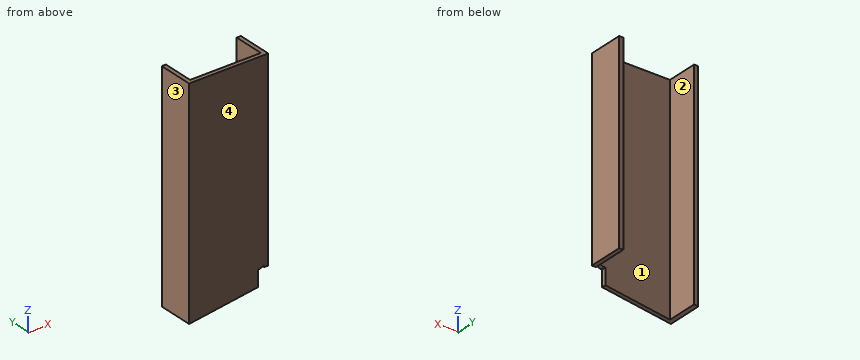
Autodesk Inventor part; units mm, degrees
ref_plane "XZ Plane" through (0, 0, 0) normal (0, 1, 0) x (-1, 0, 0)
ref_plane "XY Plane" through (0, 0, 0) normal (0, 0, 1) x (1, 0, 0)
sketch "Sketch1" plane through (0, 0, 0) normal (0, 0, 1) x (1, 0, 0)
  line L0 (10.7104, 9.7791) -> (42.7104, 9.7791)
  line L1 (42.7104, 9.7791) -> (42.7104, 24.7791)
  line L2 (10.7104, 9.7791) -> (10.7104, 24.7791)
  line L3 (8.7104, 24.7791) -> (8.7104, 7.7791)
  line L4 (8.7104, 7.7791) -> (44.7104, 7.7791)
  line L5 (44.7104, 7.7791) -> (44.7104, 24.7791)
  line L6 (8.7104, 24.7791) -> (10.7104, 24.7791)
  line L7 (42.7104, 24.7791) -> (44.7104, 24.7791)
  point P0 (0, 0)
  dimension "d0" = 32
  dimension "d1" = 15
  dimension "d2" = 15
  dimension "d3" = 2
extrude "Extrusion1" add sketch "Sketch1" along normal blind 100 and the other way blind 5
sketch "Sketch3" plane through (10.7104, 9.7791, 100) normal (0, 1, 0) x (1, 0, 0)
  line L0 (-2, 105) -> (-2, 0)
  line L1 (-2, 91.8971) -> (-2, 105)
  line L2 (32, 105) -> (34, 105)
  line L3 (34, 105) -> (-2, 91.8971)
  line L4 (-2, 105) -> (-2, 91.8971)
  line L5 (-2, 105) -> (34, 105)
  line L6 (0, 105) -> (0, 0)
  line L7 (0, 92.625) -> (0, 105)
  line L8 (34, 105) -> (-2, 99.9405)
  line L9 (34, 105) -> (70.3538, 105) construction
  line L10 (-2, 99.9405) -> (-2, 105)
  point P0 (-10.7104, 100)
  point P1 (-2, 99.9405)
  point P2 (0, 100.2216)
  dimension "d15" = 20
  dimension "d16" = 172
extrude "Extrusion4" cut sketch "Sketch3" along normal through all both and the other way through all contours L5 L6 L8 L0 | L5 L2 L8 L6
extrude "Extrusion5" cut sketch "Sketch3" along normal through all both and the other way through all contours L8 L6 L3 L0
ref_plane "Work Plane1" through (25.71, 0, 0) normal (1, 0, 0) x (0, 1, 0)
mirror "Mirror1" about plane through (25.71, 0, 0) normal (1, 0, 0) of "Extrusion5", "Extrusion4", "Extrusion1"
sketch "Sketch4" plane through (44.7104, 7.7791, 100) normal (1, 0, 0) x (0, 0, -1)
  line L0 (92.625, 2) -> (92.625, 17)
  line L1 (92.625, 17) -> (92.625, 2)
  line L2 (92.625, 2) -> (105, 2)
  line L3 (105, 17) -> (105, 0)
  line L4 (104.7189, 17) -> (0, 17)
  line L5 (105, 17) -> (93.3527, 17)
  line L6 (92.625, 2) -> (92.625, 0)
  line L7 (105, 0) -> (0, 0)
  line L8 (92.625, 0) -> (105, 0)
  line L9 (105, 0) -> (105, 2)
  line L10 (92.625, 17) -> (0, 17)
  line L11 (0, 0) -> (0, 17)
  line L12 (91.8971, 2) -> (0, 2)
  line L13 (0, 2) -> (91.8971, 2)
  point P0 (100, -7.7791)
  point P1 (95.3874, 17)
sketch "Sketch5" plane through (25.71, 0, 0) normal (1, 0, 0) x (0, 1, 0)
  line L0 (7.7791, 100) -> (24.7791, 100)
  line L1 (24.7791, 100) -> (9.7791, 100)
  line L2 (7.7791, 7.375) -> (9.7791, 7.375)
  line L3 (9.7791, 100) -> (9.7791, 7.375)
  line L4 (9.7791, 7.375) -> (24.7791, 7.375)
  line L5 (24.7791, 7.375) -> (24.7791, 100)
  line L6 (9.7791, 7.375) -> (9.7791, 100)
  point P0 (0, 0)
  dimension "d24" = 15
extrude "Extrusion7" cut sketch "Sketch5" along normal mid plane 34
extrude "Extrusion8" cut sketch "Sketch4" against normal blind 5 contours L0 L4 L5 L3 L2 | L2 L3 L7 L6
equation "\"BendRadius\" = Thickness"
equation "\"BendReliefWidth\" = Thickness"
equation "\"BendReliefDepth\" = 0.5 * Thickness"
equation "\"CornerReliefSize\" = 4 * Thickness"
equation "\"MinimumRemnant\" = 2 * Thickness"
equation "\"TransitionRadius\" = BendRadius"
equation "\"JacobiRadiusSize\" = BendRadius"
equation "\"GapSize\" = Thickness"
properties part number "outslideleft"
The model under review builds one solid part; all positions refer to its coordinate system, in mm. Face numbers are marked on the shaded views. Give positions to 0.01 mm unless a question says otherwise; leave off trailing zeros. Loops run counter-clockwise (first coordinate to the right, second up) from the corner with the lowest first, then second, coordinate; pieces in that order, holes last. Notation, with made-up numbers: (-15.5, -23.5) -> (10.5, -23.5) arc R9 ccw to (10.5, -16.5) -> close; hole circle Ø7 at (-22, -7.5). An arc over 180 degrees is marked (long way). Write each question's results on one line, items separated by ' | '.
1) Take a section at C-C, the plane x = 11.5. Give the boundary of the cut face in (y, z), plus the area to 3 significant figures.
Conclusion:
outline: (7.78, -4.33) -> (9.78, -4.33) -> (9.78, 100) -> (7.78, 100) -> close | area: 209 mm^2
2) Take a section at A-A, the plane y = 16.75. Give the boundary of the cut face in (x, z) (3 decimals).
Conclusion:
outline: (6.71, -5) -> (8.71, -4.719) -> (8.71, 100) -> (6.71, 100) -> close; (42.71, 7.375) -> (44.71, 7.375) -> (44.71, 100) -> (42.71, 100) -> close
3) Insertion check: pin 1 Ø0.8 at (x, y) = (40, 8.5) entering from -Z; pin 2 Ø3 at (x, z) = (26.5, 20.5) entering from +Y; pin 3 Ø6 at (x, y) = (38, 14) entering from +Z; pin 4 Ø0.6 at (y, z) = (9, 2) entering from +X. Each pin has a flat end and moves straight along its axis. Give the tip position at first contact, or say it passes through.
Conclusion:
pin 1: stops at z = -0.38 | pin 2: stops at y = 9.78 | pin 3: passes through | pin 4: stops at x = 39.71
4) For line 1 along X through (y, z) = (17, 9); line 2 along Y through (x, z) = (25, 39.5); line 3 along Z through (x, y) = (40, 9.5) (3 decimals), list the stretches that pass through material, from the lowest coordinate up. Write a range as from..to.
Conclusion:
line 1: x = 6.71..8.71, 42.71..44.71 | line 2: y = 7.78..9.78 | line 3: z = 7.375..100
5) Take a section at B-B, the plane z = 82. Give the boundary of the cut face in (x, y).
Conclusion:
outline: (6.71, 7.78) -> (44.71, 7.78) -> (44.71, 24.78) -> (42.71, 24.78) -> (42.71, 9.78) -> (8.71, 9.78) -> (8.71, 24.78) -> (6.71, 24.78) -> close
6) Take a section at D-D, the plane x = 15.5. Give the boundary of the cut face in (y, z), plus the area to 3 significant figures.
Conclusion:
outline: (7.78, -3.76) -> (9.78, -3.76) -> (9.78, 100) -> (7.78, 100) -> close | area: 208 mm^2
7) Draft analysis for pull direction X (two halves, no side actions). For the marked faces 1, 2, 3 and 4, state which applies: pulls with the +X half, pulls with the -X half, needs draft (parallel to the pull), parting line crosses it, or undercut.
Conclusion:
face 1: undercut | face 2: undercut | face 3: pulls with the -X half | face 4: needs draft
